Model file for the job. Use its own axes, mm. Round coordinates to 2 decimals unless told otherwise and drop trailing zeros. Write each loop counter-clockwise with the first axis right and the second up, starting at its lowest first coordinate (ties: lowest second). Pieces come first, ordered by that corner, then holes. Notation, with made-up numbers: (19.5, 11.25) - (54.5, 11.25) arc R21 ccw to (54.5, 43.25) - close; hole circle Ø4 at (37, 59). An arc over 180 degrees is marked (long way). Answer as a JSON object with one key per item and string values. Group by question number.
from build123d import *

# Parameters (mm, degrees)
SKETCH1_R           = 5.75
SKETCH1_R_2         = 1.5
BOSS_EXTRUDE1_DEPTH = 3.8
SKETCH2_OUTSIDE_W   = 16.84
SKETCH2_OUTSIDE_H   = 16.84
SKETCH2_OUTSIDE_R   = 5
CUT_EXTRUDE1_DEPTH  = 3
FILLET1_R           = 0.5


with BuildPart() as part:
    # Sketch1 → Boss-Extrude1 (new body)
    with BuildSketch(Plane(origin=(0, 0, 0), x_dir=(1, 0, 0), z_dir=(0, 1, 0))):
        with Locations(Location((0, 0, 0), (0, 0, 90))):
            Circle(SKETCH1_R)
        with Locations(Location((0, 0, 0), (0, 0, 90))):
            Circle(SKETCH1_R_2, mode=Mode.SUBTRACT)
    extrude(amount=BOSS_EXTRUDE1_DEPTH)

    # Sketch2 outside → Cut-Extrude1 (cut)
    with BuildSketch(Plane(origin=(0, 3.8, 0), x_dir=(1, 0, 0), z_dir=(0, 1, 0))):
        Rectangle(SKETCH2_OUTSIDE_W, SKETCH2_OUTSIDE_H)
        with Locations(Location((0, 0, 0), (0, 0, 270))):
            Circle(SKETCH2_OUTSIDE_R, mode=Mode.SUBTRACT)
    extrude(amount=-CUT_EXTRUDE1_DEPTH, mode=Mode.SUBTRACT)

    # Fillet1
    fillet1_edges = [part.edges().sort_by_distance(p)[0] for p in [
        (0, 3.8, -5),
    ]]
    fillet(fillet1_edges, radius=FILLET1_R)


solid = part.part
(1) Slice it at A-A (z = 0). Write the cut outline in (x, y), then the cut area to 3 significant figures.
(2) Slice it at B-B (x = 0). Write the cut outline in (y, z), then the cut area to 3 significant figures.
(3) Drill centre lines: line 1 (X direction, y = 1.3, z = 0); line 2 (Z direction, x = -0.75, y = 1.2); line 3 (X direction, y = 0.6, z = 0.25). Where is each one in solid material? Low to high. Write a range as from..to.
(4) Slice it at C-C (y = 1.25). Write the cut outline in (x, z).
(5) Pull direction Z, two halves, no side cores. Call faces 1 (the cylindrical face through (-4.88, 2.07, -1.08)), 2 (the flat face through (-2, 0.8, -5)), 3 (the cylindrical face through (-0.45, 1.87, -1.43)): pulls with the +Z half, pulls with the -Z half, needs draft (parallel to the pull), parting line crosses it, or undercut.
(6) Slice it at D-D (y = 0.65). Write the cut outline in (x, z).
Answer:
{
 "1": {"outline": "(-5.75, 0) - (-1.5, 0) - (-1.5, 3.8) - (-4.5, 3.8) arc R0.5 ccw to (-5, 3.3) - (-5, 0.8) - (-5.75, 0.8) - close; (1.5, 0) - (5.75, 0) - (5.75, 0.8) - (5, 0.8) - (5, 3.3) arc R0.5 ccw to (4.5, 3.8) - (1.5, 3.8) - close", "area": "27.7 mm²"},
 "2": {"outline": "(0, -5.75) - (0.8, -5.75) - (0.8, -5) - (3.3, -5) arc R0.5 ccw to (3.8, -4.5) - (3.8, -1.5) - (0, -1.5) - close; (0, 1.5) - (3.8, 1.5) - (3.8, 4.5) arc R0.5 ccw to (3.3, 5) - (0.8, 5) - (0.8, 5.75) - (0, 5.75) - close", "area": "27.7 mm²"},
 "3": {"line 1": "-5..-1.5, 1.5..5", "line 2": "-4.94..-1.3, 1.3..4.94", "line 3": "-5.74..-1.48, 1.48..5.74"},
 "4": {"outline": "circle Ø10 at (0, 0); hole circle Ø3 at (0, 0)"},
 "5": {"face 1": "parting line crosses it", "face 2": "needs draft", "face 3": "undercut"},
 "6": {"outline": "circle Ø11.5 at (0, 0); hole circle Ø3 at (0, 0)"}
}
